Source: CAD feature listing. Evaluate the final solid. Frame: model axes, mm. Round coordinates to 2 decimals unless told otherwise and drop trailing zeros. Loops run counter-clockwise (first coordinate to the right, second up) from the corner with the lowest first, then second, coordinate; pieces in that order, holes last.
(1) Mould query, pull axis X, two halves, no side actions, for faces 1 (the cylindrical face through (20, 20, 36)), 2 (the flat face through (25, -2, 36)), 3 (the flat face through (0, 23, 35)), 4 (the cylindrical face through (-3.45, -17.52, 39.74)). Classes: pulls with the +X half, pulls with the -X half, needs draft (parallel to the pull), parting line crosses it, or undercut.
(2) Section D-D, the plane x = 20. Return the cut outline in (y, z).
(3) Section B-B, the plane x = 6.5. Return the cut outline in (y, z).
(4) First-contact query: pin 1 Ø3 at (x, y) = (20, -22) entering from -Z; pin 2 Ø5 at (x, y) = (20, 18) entering from -Z. Flat tips, straight axial feed; report the tip coordinate or a pass-through.
(5) Section A-A, the plane z = 27. Return the cut outline in (x, y), plus the area to 3 significant figures.
(6) Material intervals for probe 1 along X at (y, z) = (18, 36.5); probe 2 along Y at (x, z) = (0, 38.75); probe 3 along Y at (x, z) = (-20, 28.5), sorted ascending.
(7) Section C-C, the plane y = 18. Return the cut outline in (x, z), plus the area to 3 significant figures.
```python
from build123d import *

# Parameters (mm, degrees)
SKETCH1_W               = 50
SKETCH1_H               = 50
SKETCH1_R               = 15.9
SKETCH1_R_2             = 2
BOSS_EXTRUDE1_DEPTH     = 48.6
CUT_EXTRUDE1_DEPTH      = 61.958674526
CUT_EXTRUDE1_DEPTH_BACK = 61.958674526
SKETCH2_R               = 31.75


with BuildPart() as part:
    # Sketch1 → Boss-Extrude1 (new body)
    with BuildSketch(Plane.XY):
        with Locations((0, -2)):
            Rectangle(SKETCH1_W, SKETCH1_H)
        with Locations((0, -2)):
            Circle(SKETCH1_R, mode=Mode.SUBTRACT)
        with Locations((-20, 18)):
            Circle(SKETCH1_R_2, mode=Mode.SUBTRACT)
        with Locations((20, 18)):
            Circle(SKETCH1_R_2, mode=Mode.SUBTRACT)
        with Locations((20, -22)):
            Circle(SKETCH1_R_2, mode=Mode.SUBTRACT)
        with Locations((-20, -22)):
            Circle(SKETCH1_R_2, mode=Mode.SUBTRACT)
    extrude(amount=BOSS_EXTRUDE1_DEPTH)

    # Sketch2 → Cut-Extrude1 (cut, two sides: drawn at the far end of the back side and taken through both)
    with BuildSketch(Plane(origin=(0, 0, 0), x_dir=(0, 0, -1), z_dir=(1, 0, 0)).offset(-CUT_EXTRUDE1_DEPTH_BACK)):
        Circle(SKETCH2_R)
    extrude(amount=CUT_EXTRUDE1_DEPTH + CUT_EXTRUDE1_DEPTH_BACK, mode=Mode.SUBTRACT)


solid = part.part
```
Output values:
1. face 1: undercut
1. face 2: pulls with the +X half
1. face 3: needs draft
1. face 4: undercut
2. outline: (-27, 16.71) arc R31.75 cw to (-24, 20.79) - (-24, 48.6) - (-27, 48.6) - close; (-20, 24.66) arc R31.75 cw to (16, 27.42) - (16, 48.6) - (-20, 48.6) - close; (20, 24.66) arc R31.75 cw to (23, 21.89) - (23, 48.6) - (20, 48.6) - close
3. outline: (-27, 16.71) arc R31.75 cw to (-16.51, 27.12) - (-16.51, 48.6) - (-27, 48.6) - close; (12.51, 29.18) arc R31.75 cw to (23, 21.89) - (23, 48.6) - (12.51, 48.6) - close
4. pin 1: passes through
4. pin 2: stops at z = 24.24
5. outline: (-25, -27) - (25, -27) - (25, -16.71) - (6.05, -16.71) arc R15.9 cw to (-6.05, -16.71) - (-25, -16.71) - close; (-25, 16.71) - (-21.52, 16.71) arc R2 cw (long way) to (-18.48, 16.71) - (18.48, 16.71) arc R2 cw (long way) to (21.52, 16.71) - (25, 16.71) - (25, 23) - (-25, 23) - close; hole circle Ø4 at (-20, -22); hole circle Ø4 at (20, -22)
5. area: 772 mm2
6. probe 1: x = -25 to -22, -18 to 18, 22 to 25
6. probe 2: y = -27 to -17.9, 13.9 to 23
6. probe 3: y = -27 to -24, -20 to -13.99, 13.99 to 16, 20 to 23
7. outline: (-25, 26.15) - (-22, 26.15) - (-22, 48.6) - (-25, 48.6) - close; (-18, 26.15) - (18, 26.15) - (18, 48.6) - (-18, 48.6) - close; (22, 26.15) - (25, 26.15) - (25, 48.6) - (22, 48.6) - close
7. area: 943 mm2
